Part model, mm, in its own coordinate system. Face numbers are marked on the shaded views. Round coordinates to 2 decimals unless told otherwise and drop trailing zeros. Loops run counter-clockwise (first coordinate to the right, second up) from the corner with the lowest first, then second, coordinate; pieces in that order, holes last.
(1) Mould opens along Z. For the marked faces 1, 2 and 3 say: +Z half, -Z half, draft (parallel to the pull), parting line (faces both ways), or undercut.
(2) Cut at D-D on y = 14.25. List the corners of the cut face in (x, z), then the cut area to 3 significant figures.
(3) Probe probe 1 along Z at (x, y) = (0, 3); probe 2 along Y at (x, z) = (-1.9, 0.1); probe 3 along X at (y, z) = (19.5, -0.7). List the from-to ranges inside material, lowest first.
(4) Cut at B-B on y = 5. List the corners of the cut face in (x, z), then the cut area to 3 significant figures.
(5) Cut at A-A on x = 0. List the corners of the cut face in (y, z), then the cut area to 3 significant figures.
(6) Cut at C-C on z = 0. List the corners of the cut face in (x, y).
from build123d import *

# Parameters (mm, degrees)
IZIM2_R               = 2
KES_EKSTR_ZYON1_DEPTH = 10
RADYUS1_R             = 0.4


with BuildPart() as part:
    # Çizim1 → Döndür1 (revolve)
    with BuildSketch(Plane.XY):
        Polygon((0, 0), (0, 30), (2, 30), (2, 20), (2.5, 20), (2.5, 0), align=None)
    revolve(axis=Axis((0, 0, 0), (0, 1, 0)))

    # Çizim2 → Kes-Ekstrüzyon1 (cut)
    with BuildSketch(Plane.XZ):
        Circle(IZIM2_R)
    extrude(amount=-KES_EKSTR_ZYON1_DEPTH, mode=Mode.SUBTRACT)

    # Radyus1
    radyus1_edges = [part.edges().sort_by_distance(p)[0] for p in [
        (-2, 0, 0),
    ]]
    fillet(radyus1_edges, radius=RADYUS1_R)


solid = part.part
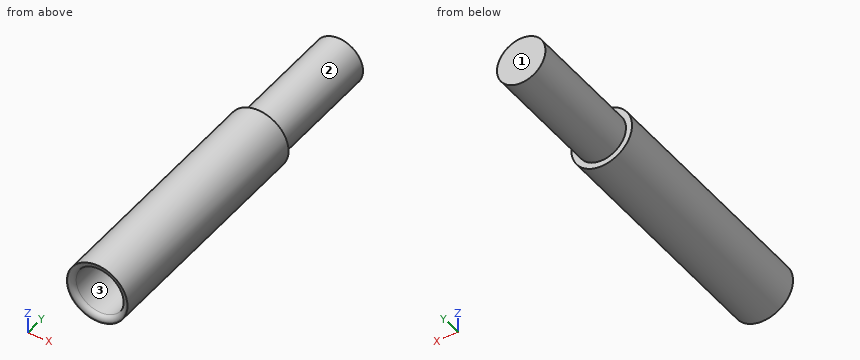
Final values:
1. face 1: draft
1. face 2: parting line
1. face 3: undercut
2. outline: circle Ø5 at (0, 0)
2. area: 19.6 mm2
3. probe 1: z = -2.5 to -2, 2 to 2.5
3. probe 2: y = 10 to 30
3. probe 3: x = -2.4 to 2.4
4. outline: circle Ø5 at (0, 0); hole circle Ø4 at (0, 0)
4. area: 7.07 mm2
5. outline: (0, -2.5) - (20, -2.5) - (20, -2) - (30, -2) - (30, 2) - (20, 2) - (20, 2.5) - (0, 2.5) - (0, 2.4) arc R0.4 ccw to (0.4, 2) - (10, 2) - (10, -2) - (0.4, -2) arc R0.4 ccw to (0, -2.4) - close
5. area: 99.9 mm2
6. outline: (-2.5, 0) - (-2.4, 0) arc R0.4 ccw to (-2, 0.4) - (-2, 10) - (2, 10) - (2, 0.4) arc R0.4 ccw to (2.4, 0) - (2.5, 0) - (2.5, 20) - (2, 20) - (2, 30) - (-2, 30) - (-2, 20) - (-2.5, 20) - close
